from build123d import *
from build123d.topology import SkipClean

# Parameters (mm, degrees)
SKETCH1_R                = 18.415
BOSS_EXTRUDE1_DEPTH      = 63.5
BOSS_EXTRUDE4_DEPTH      = 12.7
SKETCH9_R                = 1.778
CUT_EXTRUDE2_DEPTH       = 25.4
BOSS_EXTRUDE5_DEPTH      = 1.27
BOSS_EXTRUDE5_DEPTH_BACK = 1.27
CUT_EXTRUDE3_DEPTH       = 15.24
CUT_EXTRUDE4_START       = -12.7
CUT_EXTRUDE4_DEPTH       = 12.7
CIRPATTERN1_COUNT        = 4


with BuildPart() as part:
    # Sketch1 → Boss-Extrude1 (new body)
    with BuildSketch(Plane.XY):
        Circle(SKETCH1_R)
    extrude(amount=BOSS_EXTRUDE1_DEPTH)

    # Sketch8 → Boss-Extrude4 (add)
    with BuildSketch(Plane.XY):
        with BuildLine():
            Line((-14.438397591, 11.43), (-32.218397591, 11.43))
            Line((-32.218397591, 11.43), (-32.218397591, -11.43))
            Line((-32.218397591, -11.43), (-14.438397591, -11.43))
            ThreePointArc((-14.438397591, -11.43), (-18.415, 0), (-14.438397591, 11.43))
        make_face()
    boss_extrude4 = extrude(amount=BOSS_EXTRUDE4_DEPTH)

    # Sketch9 → Cut-Extrude2 (cut)
    with BuildSketch(Plane.XZ.offset(11.43)):
        with Locations(Location((-24.598397591, 6.35, 0), (0, 0, 270))):
            Circle(SKETCH9_R)
    cut_extrude2 = extrude(amount=-CUT_EXTRUDE2_DEPTH, mode=Mode.SUBTRACT)

    # Sketch13 → Boss-Extrude5 (add, two sides: drawn at the far end of the back side and taken through both)
    with BuildSketch(Plane(origin=(0, 0, 0), x_dir=(0, 0, -1), z_dir=(1, 0, 0)).offset(-BOSS_EXTRUDE5_DEPTH_BACK)):
        with BuildLine():
            Line((-63.5, 6.35), (-63.5, -6.35))
            ThreePointArc((-63.5, -6.35), (-69.85, 0), (-63.5, 6.35))
        make_face()
    extrude(amount=BOSS_EXTRUDE5_DEPTH + BOSS_EXTRUDE5_DEPTH_BACK)

    # Sketch14 → Cut-Extrude3 (cut)
    with BuildSketch(Plane(origin=(1.27, 0, 0), x_dir=(0, 0, -1), z_dir=(1, 0, 0))):
        with BuildLine():
            Line((-63.5, 3.81), (-63.5, -3.81))
            ThreePointArc((-63.5, -3.81), (-67.31, 0), (-63.5, 3.81))
        make_face()
    extrude(amount=-CUT_EXTRUDE3_DEPTH, mode=Mode.SUBTRACT)

    # Sketch15 → Cut-Extrude4 (cut)
    with SkipClean():  # the faces are left unmerged after this step: merging them gives an invalid solid
        with BuildSketch(Plane.XY.offset(12.7).offset(CUT_EXTRUDE4_START)):
            with BuildLine():
                Line((-17.285535138, 6.35), (-32.218397591, 6.35))
                Line((-32.218397591, 6.35), (-32.218397591, -6.35))
                Line((-32.218397591, -6.35), (-17.285535138, -6.35))
                ThreePointArc((-17.285535138, -6.35), (-18.415, 0), (-17.285535138, 6.35))
            make_face()
        cut_extrude4 = extrude(amount=CUT_EXTRUDE4_DEPTH, mode=Mode.SUBTRACT)

    # CirPattern1: Boss-Extrude4, Cut-Extrude2, Cut-Extrude4 ×4 about axis
    with SkipClean():  # the faces are left unmerged after this step: merging them gives an invalid solid
        cirpattern1_axis = Axis((0, 0, 0), (0, 0, 1))
        add([boss_extrude4.rotate(cirpattern1_axis, i * 360 / CIRPATTERN1_COUNT) for i in range(1, CIRPATTERN1_COUNT)])
        add([cut_extrude2.rotate(cirpattern1_axis, i * 360 / CIRPATTERN1_COUNT) for i in range(1, CIRPATTERN1_COUNT)], mode=Mode.SUBTRACT)
        add([cut_extrude4.rotate(cirpattern1_axis, i * 360 / CIRPATTERN1_COUNT) for i in range(1, CIRPATTERN1_COUNT)], mode=Mode.SUBTRACT)


solid = part.part
Input: part model. Units: mm. Frame: model coordinates. A direction names the side the tool comes from. Round coordinates to 2 decimals unless told otherwise and drop trailing zeros. Order: outer loops, then holes, each group sorted by start corner. A loop starts at its lowest first (then second) coordinate and runs counter-clockwise, first axis right, second up. Notation, with made-up numbers: (-34, -27) - (22, -27) arc R10 cw to (22, -17) - close; hole circle Ø3 at (79, 88). An arc over 180 degrees is marked (long way). Answer as a JSON object with one key per item and string values. Group by question number.
(1) Cut plane C-C (z = 6.35). Count the separate pieces of the cut face and the enclosed holes in it, then the cut area to 3 significant figures.
(2) Pin query (flat end, axial travel): P1, Ø1.5, axis at x = -5, y = -16, coming from the -Z side; P2, Ø5, axis at x = 0, z = 8, coming from the -Y side (3 decimals); P3, Ø2.5, axis at x = -23.5, y = 9, coming from the +Z side; P4, Ø4, axis at y = 25.5, z = 8, coming from the -X side. Return the tip coordinate at first contact, or that it passes through.
(3) Cut plane B-B (x = 0). Return loops of the section in (y, z) (3 decimals).
(4) Draft query along Z for faces 1 (the face through (11.43, -23, 5)), 2 (the face through (-9, 23, 12.7)), 3 (the face through (-8.854, -22.836, 6.581)). Return one class per face: released by +Z, released by -Z, zero draft, split by the parting line, or undercut.
(5) Cut plane A-A (y = 0). Return loops of the section in (x, z) (3 decimals).
(6) Cut plane D-D (x = 9). Return loops of the section in (y, z).
(7) Reachability of faces 4 (the face through (-1.27, 0, 68)), 5 (the face through (27, 6.35, 6)), 6 (the face through (-11.43, 23, 5)), 7 (the face through (6.35, -27, 6)), 8 (the face through (9, 23, 12.7)) from +Z, -Z, +X, -X, +Y, -Y: full face, straight path, thin tool, end or side. Return the list, or none.
(8) Material intervals for probe 1 along X at (y, z) = (10.25, 6.35); probe 2 along X at (y, z) = (-24, 4), sorted ascending. Write a range as from..to.
Here are the results:
{
 "1": {"separate pieces": "9", "enclosed holes": "0", "area": "1,580 mm^2"},
 "2": {"P1": "stops at z = 0", "P2": "stops at y = -18.415", "P3": "stops at z = 12.7", "P4": "stops at x = -11.43"},
 "3": {"outline": "(-18.415, 0) - (18.415, 0) - (18.415, 63.5) - (6.35, 63.5) arc R6.35 ccw to (-6.35, 63.5) - (-18.415, 63.5) - close; hole (-3.81, 63.5) - (3.81, 63.5) arc R3.81 ccw to start"},
 "4": {"face 1": "zero draft", "face 2": "released by +Z", "face 3": "undercut"},
 "5": {"outline": "(-18.415, 0) - (18.415, 0) - (18.415, 63.5) - (-18.415, 63.5) - close; (-1.27, 67.31) - (1.27, 67.31) - (1.27, 69.85) - (-1.27, 69.85) - close"},
 "6": {"outline": "(-32.22, 0) - (32.22, 0) - (32.22, 12.7) - (16.07, 12.7) - (16.07, 63.5) - (-16.07, 63.5) - (-16.07, 12.7) - (-32.22, 12.7) - close; hole circle Ø3.56 at (-24.6, 6.35); hole circle Ø3.56 at (24.6, 6.35)"},
 "7": {"face 4": "+Z, -X, +Y, -Y", "face 5": "+Z, -Z, +X", "face 6": "+Z, -Z, -X, +Y", "face 7": "+Z, -Z, -Y", "face 8": "+Z, +X, +Y"},
 "8": {"probe 1": "x = -32.22..-26.38, -22.82..22.82, 26.38..32.22", "probe 2": "x = -11.43..-6.35, 6.35..11.43"}
}
